Input: part model. Units: mm. Frame: model coordinates. A direction names the side the tool comes from. Give positions to 0.01 mm unless a question says otherwise; leave off trailing zeros. Write each loop counter-clockwise with the first axis right and the second up, starting at its lowest first coordinate (ties: lowest second). Pieces come first, ordered by that corner, then holes. Notation, with made-up numbers: (65.25, -14) -> (87.25, -14) arc R26 ccw to (87.25, 15) -> close; hole circle Ø1 at (-12, 39.25). An arc over 180 degrees is marked (long way). Return JSON: item names as keys, results as strings. Group by question number.
Item 1: Section B-B, the plane x = 7.75. Return loops of the section in (y, z), then the cut area to 3 significant figures.
Item 2: Set-up query: faces 1 (the face through (-4, 16, 8)), 2 (the face through (8, 16, 4)), 3 (the face through (7, 17, 7)), 4 (the face through (0, 8, -8.5)), 5 (the face through (4.301, 16.014, 6.785)). Return all of +Z, -Z, +X, -X, +Y, -Y with unobstructed straight access to the full face (end or side cutting, diameter ignored); none if empty.
Item 3: Section A-A, the plane y = 13. Return loops of the section in (x, z).
Item 4: Section C-C, the plane z = -0.5. Return loops of the section in (x, y).
Item 5: Line query: line 1 (X direction, y = 2.75, z = 5.75); line 2 (Z direction, x = -7.5, y = 15.25). Output: solid intervals per line, ascending. Write a range as [from, to].
Item 6: Pin query (flat end, axial travel): P1, Ø2, axis at x = 6, z = 5.5, coming from the -Y side; P2, Ø2, axis at x = -2, z = 2.5, coming from the +Y side; P3, Ø1, axis at x = -0.5, z = 7.5, coming from the +Y side. Return the tip coordinate at first contact, or that it passes through.
Item 7: Section D-D, the plane x = -4.25. Return loops of the section in (y, z), then the cut area to 3 significant figures.
Autodesk Inventor part; units mm, degrees
ref_plane "YZ Plane" through (0, 0, 0) normal (1, 0, 0) x (0, 1, 0)
ref_plane "XZ Plane" through (0, 0, 0) normal (0, 1, 0) x (-1, 0, 0)
ref_plane "XY Plane" through (0, 0, 0) normal (0, 0, 1) x (1, 0, 0)
sketch "Sketch1" plane through (0, 0, 0) normal (0, 1, 0) x (-1, 0, 0)
  line L0 (8.5, 8.5) -> (-8.5, 8.5)
  line L1 (-8.5, 8.5) -> (-8.5, -8.5)
  line L2 (-8.5, -8.5) -> (8.5, -8.5)
  line L3 (8.5, -8.5) -> (8.5, 8.5)
  line L4 (6.5, 6.5) -> (-6.5, 6.5) construction
  line L5 (-6.5, 6.5) -> (-6.5, -6.5) construction
  line L6 (-6.5, -6.5) -> (6.5, -6.5) construction
  line L7 (6.5, -6.5) -> (6.5, 6.5) construction
  point P0 (0, 0)
  point P1 (8.5, 0)
  point P2 (0, -6.5)
  point P3 (0, -8.5)
  point P4 (6.5, 0)
  dimension "d0" = 13
  dimension "d1" = 13
  dimension "d2" = 17
extrude "Extrusion1" add sketch "Sketch1" along normal blind 17
shell "Shell1" thickness 2 removed faces 1 at (2.8333, 17, 2.8333)
sketch "Sketch2" plane through (0, 17, 0) normal (0, 1, 0) x (1, 0, 0)
  line L0 (6, -4) -> (8.5, -4)
  line L1 (4, -6) -> (4, -8.5)
  line L2 (0, -12.5225) -> (0, 10.2466) construction
  line L3 (-9.8637, 0) -> (11.1563, 0) construction
  line L4 (4, -8.5) -> (0, -8.5)
  line L5 (0, -8.5) -> (4, -8.5) construction
  line L6 (-8.5, -8.5) -> (8.5, -8.5) construction
  line L7 (6, 4) -> (8.5, 4)
  line L8 (8.5, 4) -> (8.5, 0)
  line L9 (4, 6) -> (4, 8.5)
  line L10 (4, 8.5) -> (0, 8.5)
  line L11 (8.5, -4) -> (8.5, 4)
  line L12 (-6, -4) -> (-8.5, -4)
  line L13 (-4, -6) -> (-4, -8.5)
  line L14 (-4, -8.5) -> (0, -8.5)
  line L15 (-4, 8.5) -> (0, 8.5)
  line L16 (-4, 6) -> (-4, 8.5)
  line L17 (-6, 4) -> (-8.5, 4)
  line L18 (-8.5, 4) -> (-8.5, 0)
  line L19 (-8.5, -4) -> (-8.5, 4)
  arc A0 (-4, -6) -> (-6, -4) centre (-6, -6) ccw
  arc A1 (-6, 4) -> (-4, 6) centre (-6, 6) ccw
  arc A2 (4, 6) -> (6, 4) centre (6, 6) ccw
  arc A3 (6, -4) -> (4, -6) centre (6, -6) ccw
  point P0 (0, 0)
  point P1 (4, -4)
  point P2 (4, 4)
  point P3 (-4, -4)
  point P4 (-11.1563, 0)
  point P5 (-4, 4)
  dimension "d6" = 4
  dimension "d7" = 4
  dimension "d8" = 2
extrude "Extrusion2" cut sketch "Sketch2" against normal blind 2
fillet "Fillet1" radius 1 8 edges at (-6.5, 16, 4) (-4, 16, 6.5) (-6.5, 16, -4) (-4, 16, -6.5) (4, 16, -6.5) (6.5, 16, -4) (6.5, 16, 4) (4, 16, 6.5)
equation "\"d3\" = d2"
equation "\"d7\" = d6"
properties part number "reference_magnet_box"
Answer below:
{
 "1": {"outline": "(0, -8.5) -> (17, -8.5) -> (17, -4) -> (15, -4) -> (15, 4) -> (17, 4) -> (17, 8.5) -> (0, 8.5) -> close", "area": "273 mm2"},
 "2": {"face 1": "+Z, -Z, +Y", "face 2": "+X, -X, +Y", "face 3": "+Z, -Z, +X, -X, +Y", "face 4": "-Z, +X, -X, +Y, -Y", "face 5": "+Y"},
 "3": {"outline": "(-8.5, -8.5) -> (8.5, -8.5) -> (8.5, 8.5) -> (-8.5, 8.5) -> close; hole (-6.5, -6.5) -> (6.5, -6.5) -> (6.5, 6.5) -> (-6.5, 6.5) -> close"},
 "4": {"outline": "(-8.5, 0) -> (8.5, 0) -> (8.5, 15) -> (6.5, 15) -> (6.5, 2) -> (-6.5, 2) -> (-6.5, 15) -> (-8.5, 15) -> close"},
 "5": {"line 1": "x = [-8.5, -6.5], [6.5, 8.5]", "line 2": "z = [-8.5, -4], [4, 8.5]"},
 "6": {"P1": "stops at y = 0", "P2": "stops at y = 2", "P3": "stops at y = 15"},
 "7": {"outline": "(0, -8.5) -> (17, -8.5) -> (17, -6.84) -> (15, -6.84) -> (15, -6.5) -> (2, -6.5) -> (2, 6.5) -> (15, 6.5) -> (15, 6.84) -> (17, 6.84) -> (17, 8.5) -> (0, 8.5) -> close", "area": "92.6 mm2"}
}
